Check sheet for the modelled part. Datum: model origin and axes. Units: mm. A direction names the side the tool comes from. Give positions to 0.01 mm unless a question says otherwise; leave off trailing zeros. Order: outer loops, then holes, each group sorted by start corner. A loop starts at its lowest first (then second) coordinate and runs counter-clockwise, first axis right, second up.
Item 1: Sectioned sample at C-C on z = 0.25. Count the separate pieces of the cut face and the enclosed holes in it, and give its area (3 significant figures).
Item 2: Sectioned sample at A-A on x = 101.6. Record the boundary of the cut face in (y, z) (3 decimals), and give its area (3 significant figures).
Item 3: Release check for a two-part mould opening along Y. For faces 4 (the cylindrical face through (-1.178, 124.735, -0.044)), 5 (the flat face through (157.162, 0, 0)), 6 (the flat face through (102, 12.7, 0)) record: released by +Y, released by -Y, zero draft, split by the parting line, or undercut.
Item 4: Access from +Z, -Z, +X, -X, +Y, -Y to the whole of each face (thin tool, end or side, straight path). Record for faces 1 (the cylindrical face through (155.35, -10.79, -0.04)), 2 (the flat face through (0, 25.4, 0)), 3 (the flat face through (12.7, 103, 0)).
Item 5: Material ranges on line 1 along Y through (x, z) = (0, -1.5); line 2 along X through (y, z) = (0, 0.5); line 3 along Y through (x, z) = (127, -1.5), recorded low to high.
Item 6: Gauge pin test, flat ends, axial feed: P1, Ø1.9, axis at y = 43.5, z = 0.5, coming from the +X side; P2, Ø6.5, axis at x = 0, y = 101.6, coming from the -Z side (3 decimals); P3, Ø1.9, axis at y = 110, z = 1, coming from the +X side; P4, Ø1.5, axis at x = 77.5, z = 0.5, coming from the +Y side. Record the tip position at first contact, or that the pin passes through.
Item 7: Sectioned sample at B-B on y = 79. Record the boundary of the cut face in (x, z) (1 decimal), and give its area (3 significant figures).
Autodesk Inventor part; units mm, degrees
ref_plane "Work Plane2" through (0, 0, 0) normal (-0.7071, 0.7071, 0) x (0, 0, 1)
ref_plane "XY Plane" through (0, 0, 0) normal (0, 0, 1) x (1, 0, 0)
ref_plane "Work Plane2" through (0, 0, 0) normal (-0.7071, 0.7071, 0) x (0, 0, 1)
sketch "Sketch1" plane through (-160.3375, 44.45, 0) normal (0, 0, 1) x (1, 0, 0)
  line L0 (311.15, -57.15) -> (160.3375, -57.15)
  arc A0 (311.15, -57.15) -> (317.5, -50.8) centre (311.15, -50.8) ccw
  line L1 (317.5, -38.1) -> (317.5, -50.8)
  arc A1 (317.5, -38.1) -> (311.15, -31.75) centre (311.15, -38.1) ccw
  line L2 (214.3125, -31.75) -> (311.15, -31.75)
  line L3 (173.0375, 106.3625) -> (173.0375, 9.525)
  arc A2 (173.0375, 106.3625) -> (166.6875, 112.7125) centre (166.6875, 106.3625) ccw
  line L4 (153.9875, 112.7125) -> (166.6875, 112.7125)
  arc A3 (153.9875, 112.7125) -> (147.6375, 106.3625) centre (153.9875, 106.3625) ccw
  line L5 (147.6375, -44.45) -> (147.6375, 106.3625)
  arc A4 (147.6375, -44.45) -> (160.3375, -57.15) centre (160.3375, -44.45) ccw
  line L6 (160.3375, -94.5418) -> (160.3375, 148.7892) construction
  line L7 (110.2457, -44.45) -> (353.5767, -44.45) construction
  arc A5 (173.0375, 9.525) -> (214.3125, -31.75) centre (214.3125, 9.525) ccw
  dimension "d1" = 169.8625
  dimension "d2" = 12.7
  dimension "d5" = 25.4
  dimension "d6" = 25.4
  dimension "d8" = 6.35
  dimension "d44" = 41.275
extrude "Extrusion1" add sketch "Sketch1" along normal mid plane 6.35
sketch "Sketch2" plane through (-160.3375, 44.45, 3.175) normal (0, 0, 1) x (1, 0, 0)
  line L0 (160.3375, -91.1225) -> (160.3375, 146.685) construction
  line L1 (113.665, -44.45) -> (351.4725, -44.45) construction
  line L2 (317.5, -50.8) -> (317.5, -38.1) construction
  point P0 (160.3375, -44.45)
  point P1 (312.7375, -44.45)
  dimension "d13" = 152.4
hole "Hole1" at (152.4, 0, 3.175) direction (0, 0, -1) diameter 5.1054 end through all
pattern_linear "Rectangular Pattern1" count 3 spacing 25.4 along (-1, 0, 0) of "Hole1"
sketch "Sketch4" plane through (-160.3375, 44.45, 3.175) normal (0, 0, 1) x (1, 0, 0)
  point P0 (160.3375, -44.45)
  point P1 (160.3375, -44.45)
hole "Hole2" at (0, 0, 3.175) direction (0, 0, -1) diameter 5.1054 end through all
mirror "Mirror1" about plane through (0, 0, 0) normal (-0.7071, 0.7071, 0) of "Hole1", "Rectangular Pattern1"
sketch "Sketch5" plane through (-160.3375, 44.45, 3.175) normal (0, 0, 1) x (1, 0, 0)
  line L0 (163.5125, 38.1) -> (157.1625, 38.1)
  line L1 (155.575, 36.5125) -> (155.575, -17.4625)
  line L2 (157.1625, -19.05) -> (163.5125, -19.05)
  line L3 (165.1, -17.4625) -> (165.1, 36.5125)
  line L4 (160.3375, -91.1225) -> (160.3375, 146.685) construction
  arc A0 (165.1, 36.5125) -> (163.5125, 38.1) centre (163.5125, 36.5125) ccw
  arc A1 (157.1625, 38.1) -> (155.575, 36.5125) centre (157.1625, 36.5125) ccw
  arc A2 (155.575, -17.4625) -> (157.1625, -19.05) centre (157.1625, -17.4625) ccw
  arc A3 (163.5125, -19.05) -> (165.1, -17.4625) centre (163.5125, -17.4625) ccw
  point P0 (160.3375, -44.45)
  point P1 (155.575, -19.05)
  point P2 (155.575, 38.1)
  point P3 (165.1, -19.05)
  dimension "d45" = 9.525
  dimension "d46" = 25.4
  dimension "d47" = 57.15
  dimension "d48" = 1.5875
extrude "Extrusion3" cut sketch "Sketch5" against normal up to surface (6.35 mm away)
properties part number "PLATE,CLAMP,MK4i,Swerve,CUSTOM,FRC2026" material "Aluminum 7075"
Report:
1. separate pieces: 1
1. enclosed holes: 8
1. area: 7,590 mm2
2. outline: (-12.7, -3.175) - (-2.553, -3.175) - (-2.553, 3.175) - (-12.7, 3.175) - close; (2.553, -3.175) - (12.7, -3.175) - (12.7, 3.175) - (2.553, 3.175) - close
2. area: 129 mm2
3. face 4: undercut
3. face 5: zero draft
3. face 6: released by +Y
4. face 1: +Z, -Z, +X, -Y
4. face 2: +Z, -Z
4. face 3: +Z, -Z, +X, +Y
5. line 1: y = -12.7 to -2.55, 2.55 to 25.4, 82.55 to 99.05, 104.15 to 124.45, 129.55 to 149.85, 154.95 to 157.16
5. line 2: x = -12.7 to -2.55, 2.55 to 99.05, 104.15 to 124.45, 129.55 to 149.85, 154.95 to 157.16
5. line 3: y = -12.7 to -2.55, 2.55 to 12.7
6. P1: stops at x = 14.31
6. P2: stops at z = -3.175
6. P3: stops at x = 12.7
6. P4: stops at y = 12.7
7. outline: (-12.7, -3.2) - (-4.8, -3.2) - (-4.8, 3.2) - (-12.7, 3.2) - close; (4.8, -3.2) - (12.7, -3.2) - (12.7, 3.2) - (4.8, 3.2) - close
7. area: 101 mm2
